from build123d import *

# Parameters (mm, degrees)
SKETCH1_R           = 11.5824
BOSS_EXTRUDE1_DEPTH = 42.9514
SKETCH2_R           = 6.7437
SKETCH2_R_2         = 4.6355
BOSS_EXTRUDE2_DEPTH = 0.6604
SKETCH3_R           = 0.9525
BOSS_EXTRUDE3_DEPTH = 2.2352
CIRPATTERN1_COUNT   = 3
SKETCH4_R           = 3.6703
SKETCH4_R_2         = 2.4511
BOSS_EXTRUDE4_DEPTH = 18.923
CHAMFER1_SIZE       = 0.79375
SKETCH5_R           = 1.36525
BOSS_EXTRUDE5_DEPTH = 10.16
BOSS_EXTRUDE6_DEPTH = 27.432


with BuildPart() as part:
    # Sketch1 → Boss-Extrude1 (new body)
    with BuildSketch(Plane(origin=(0, 0, 0), x_dir=(1, 0, 0), z_dir=(0, 1, 0))):
        with Locations(Location((0, 0, 0), (0, 0, 270))):
            Circle(SKETCH1_R)
    extrude(amount=BOSS_EXTRUDE1_DEPTH)

    # Sketch2 → Boss-Extrude2 (add)
    with BuildSketch(Plane(origin=(0, 42.9514, 0), x_dir=(1, 0, 0), z_dir=(0, 1, 0))):
        with Locations(Location((0, 0, 0), (0, 0, 270))):
            Circle(SKETCH2_R)
        with Locations(Location((0, 0, 0), (0, 0, 270))):
            Circle(SKETCH2_R_2, mode=Mode.SUBTRACT)
    extrude(amount=BOSS_EXTRUDE2_DEPTH)

    # Sketch3 → Boss-Extrude3 (add)
    with BuildSketch(Plane(origin=(0, 42.9514, 0), x_dir=(1, 0, 0), z_dir=(0, 1, 0))):
        with Locations(Location((0, 9.398, 0), (0, 0, 270))):
            Circle(SKETCH3_R)
    boss_extrude3 = extrude(amount=BOSS_EXTRUDE3_DEPTH)

    # CirPattern1: Boss-Extrude3 ×3 about axis
    cirpattern1_axis = Axis((0, 0, 0), (0, 1, 0))
    for i in range(1, CIRPATTERN1_COUNT):
        add(boss_extrude3.rotate(cirpattern1_axis, i * 360 / CIRPATTERN1_COUNT))

    # Sketch4 → Boss-Extrude4 (add)
    with BuildSketch(Plane.XY):
        with Locations((-7.9121, 37.8333)):
            Circle(SKETCH4_R)
        with Locations((-7.9121, 37.8333)):
            Circle(SKETCH4_R_2, mode=Mode.SUBTRACT)
    extrude(amount=-BOSS_EXTRUDE4_DEPTH)

    # Chamfer1
    chamfer1_edges = [part.edges().sort_by_distance(p)[0] for p in [
        (-11.5824, 37.8333, -18.923),
    ]]
    chamfer(chamfer1_edges, length=CHAMFER1_SIZE)

    # Sketch5 → Boss-Extrude5 (add)
    with BuildSketch(Plane.XZ):
        with Locations(Location((4.318, 4.318, 0), (0, 0, 90))):
            Circle(SKETCH5_R)
    extrude(amount=BOSS_EXTRUDE5_DEPTH)

    # Sketch7 → Boss-Extrude6 (add)
    with BuildSketch(Plane(origin=(0, 32.7914, 0), x_dir=(1, 0, 0), z_dir=(0, 1, 0))):
        Polygon((0, 0), (0, -11.5824), (8.001, -11.5824), (8.494294737, -12.192), (9.865894737, -12.192), align=None)
        Polygon((-8.494294737, -12.192), (-8.001, -11.5824), (0, -11.5824), (0, 0), (-9.865894737, -12.192), align=None)
    extrude(amount=-BOSS_EXTRUDE6_DEPTH)


solid = part.part
Can you work these out from the model? Positions are in its coordinate system, mm. A direction names the side the tool comes from. Give positions to 0.01 mm unless a question says otherwise; leave off trailing zeros. Order: outer loops, then holes, each group sorted by start corner. A loop starts at its lowest first (then second) coordinate and runs counter-clockwise, first axis right, second up. Notation, with made-up numbers: (39.25, -35.5) - (63.25, -35.5) arc R34 ccw to (63.25, 3.5) - close; hole circle Ø7 at (84.5, 17.5). An arc over 180 degrees is marked (long way). Write each question's results on one line, items separated by ' | '.
1) Suppose I cut it at A-A, the plane x = 1.5. Write out the boundary of the cut face in (y, z).
Final values:
outline: (0, -11.48) - (42.95, -11.48) - (42.95, -6.57) - (43.61, -6.57) - (43.61, -4.39) - (42.95, -4.39) - (42.95, 4.39) - (43.61, 4.39) - (43.61, 6.57) - (42.95, 6.57) - (42.95, 11.48) - (32.79, 11.48) - (32.79, 11.58) - (5.36, 11.58) - (5.36, 11.48) - (0, 11.48) - close
2) Suppose I cut it at B-B, the plane y = 26.5. Write out the boundary of the cut face in (x, z).
Final values:
outline: (-9.87, 12.19) - (-7.29, 9) arc R11.58 ccw (long way) to (7.29, 9) - (9.87, 12.19) - (8.49, 12.19) - (8, 11.58) - (-8, 11.58) - (-8.49, 12.19) - close
3) If we mould it in two halves opening along Z, with no side actions, what happens to faces 1 (the face through (0, 19, 11.582)), 2 (the face through (1.392, 43.277, 4.421)), 3 (the face through (-6, 32.791, 11))? For each: pulls with the +Z half, pulls with the -Z half, needs draft (parallel to the pull), parting line crosses it, or undercut.
Final values:
face 1: pulls with the +Z half | face 2: undercut | face 3: needs draft
4) Suppose I cut it at C-C, the plane z = -9. Write out the boundary of the cut face in (x, y).
Final values:
outline: (-7.29, 0) - (7.29, 0) - (7.29, 42.95) - (0.87, 42.95) - (0.87, 45.19) - (-0.87, 45.19) - (-0.87, 42.95) - (-7.29, 42.95) - (-7.29, 41.45) arc R3.67 ccw (long way) to (-7.29, 34.22) - close; hole (-7.29, 35.46) - (-7.29, 40.2) arc R2.45 ccw (long way) to start
5) I'm going to push flat-ended pins straight in: pin 1 Ø1.5 at (x, y) = (5, 7) entering from +Z; pin 2 Ø8.5 at (x, z) = (0, 0) entering from -Y; pin 3 Ø2 at (x, y) = (-7, 12) entering from -Z; pin 4 Ø1 at (y, z) = (13.5, -12.5) entering from +X. Where does each tip first touch, or does it pass through?
Final values:
pin 1: stops at z = 11.58 | pin 2: stops at y = 0 | pin 3: stops at z = -9.91 | pin 4: passes through
6) Suppose I cut it at D-D, the plane z = -13.5. Write out the boundary of the cut face in (x, y), then the cut area to 3 significant figures.
Final values:
outline: circle Ø7.34 at (-7.91, 37.83); hole circle Ø4.9 at (-7.91, 37.83) | area: 23.4 mm^2
7) Please list where these lines run through material, in increasing order: line 1 along Y through (x, z) = (-1.75, 6); line 2 along Y through (x, z) = (3, -3); line 3 along X through (y, z) = (43.3, 0). Write a range as [from, to].
Final values:
line 1: y = [0, 43.61] | line 2: y = [0, 42.95] | line 3: x = [-6.74, -4.64], [4.64, 6.74]
8) On a 3-axis mill with a long thin cutter (end or side, diameter ignored), from which of +Z, -Z, +X, -X, +Y, -Y can I reach the whole of each face in a straight line? I mean faces 4 (the face through (8.594, 19.267, 10.62)), 5 (the face through (6, 32.791, 11)), 6 (the face through (0.04, 44.05, -10.35)), 7 (the face through (-6, 5.359, 11)). Say none if no direction works.
Final values:
face 4: +X, +Y, -Y | face 5: +Z, +X, +Y | face 6: +Y | face 7: +Z, -X, -Y
